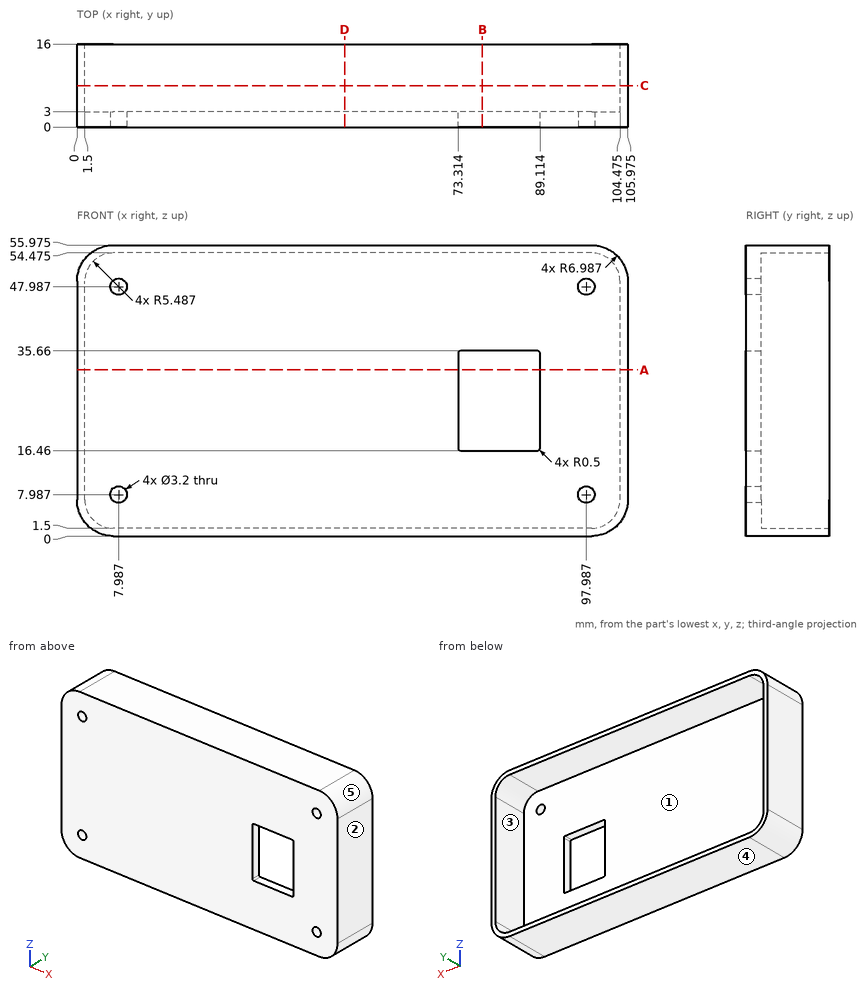
Design review of the part shown in the three views and the two pictorial views. Dimensions are in mm from the part's minimum x, y and z. A direction names the side the tool comes from. Coordinates: 2 decimals unless noted, no trailing zeros. Order: outer loops, then holes, each group sorted by start corner. A loop starts at its lowest first (then second) coordinate and runs counter-clockwise, first axis right, second up. Notation, with made-up numbers: (55.25, 55.25) - (98.25, 55.25) arc R25 cw to (98.25, 83.25) - close; hole circle Ø8 at (13.25, 28.5). An arc over 180 degrees is marked (long way). One line per question, with ' | ' between items.
Q1. For the marked faces 1 and 2, list the 3-axis set-ups (+Z, -Z, +X, -X, +Y, -Y) from which the entire face can be reached by the end or side of a thin tool; tool diameter is ignored.
Answer key:
face 1: +Y | face 2: +Z, -Z, +X, +Y, -Y
Q2. The part is to be moulded in two halves that separate along X. For the marked faces 3, 4 and 5, say which applies: +X half, -X half, draft (parallel to the pull), parting line (faces both ways), or undercut.
Answer key:
face 3: undercut | face 4: draft | face 5: +X half
Q3. Consider section B-B, the plane x = 78. Give the boundary of the cut face in (y, z) (1 decimal), then the cut area to 3 significant figures.
Answer key:
outline: (0, 0) - (16, 0) - (16, 1.5) - (3, 1.5) - (3, 16.5) - (0, 16.5) - close; (0, 35.7) - (3, 35.7) - (3, 54.5) - (16, 54.5) - (16, 56) - (0, 56) - close | area: 149 mm2
Q4. Clearance check with flat-ended pins moving along their axes: pin 1 Ø1.9 at (x, z) = (97.99, 7.99) entering from -Y; pin 2 Ø2 at (x, z) = (92, 9) entering from +Y. State where each tip first meets the part, or that it passes through.
Answer key:
pin 1: passes through | pin 2: stops at y = 3
Q5. Consider section D-D, the plane x = 51.5. Give the boundary of the cut face in (y, z) (1 decimal), then the cut area to 3 significant figures.
Answer key:
outline: (0, 0) - (16, 0) - (16, 1.5) - (3, 1.5) - (3, 54.5) - (16, 54.5) - (16, 56) - (0, 56) - close | area: 207 mm2
Q6. To check wall thickness, follow line 1 along X through (y, z) = (0.5, 28) (1 decimal); line 2 along X through (y, z) = (14.25, 36.5) (1 decimal); line 3 along Z through (x, y) = (66, 9) (1 decimal). State the ranges of each line that lie inside material, in increasing order.
Answer key:
line 1: x = 0 to 73.3, 89.1 to 106 | line 2: x = 0 to 1.5, 104.5 to 106 | line 3: z = 0 to 1.5, 54.5 to 56
Q7. Consider section C-C, the plane y = 8. Give the boundary of the cut face in (x, z) (1 decimal).
Answer key:
outline: (0, 7) arc R7 ccw to (7, 0) - (99, 0) arc R7 ccw to (106, 7) - (106, 49) arc R7 ccw to (99, 56) - (7, 56) arc R7 ccw to (0, 49) - close; hole (1.5, 7) arc R5.5 ccw to (7, 1.5) - (99, 1.5) arc R5.5 ccw to (104.5, 7) - (104.5, 49) arc R5.5 ccw to (99, 54.5) - (7, 54.5) arc R5.5 ccw to (1.5, 49) - close
Q8. Consider section A-A, the plane z = 32. Give the boundary of the cut face in (x, y) (1 decimal).
Answer key:
outline: (0, 0) - (73.3, 0) - (73.3, 3) - (1.5, 3) - (1.5, 16) - (0, 16) - close; (89.1, 0) - (106, 0) - (106, 16) - (104.5, 16) - (104.5, 3) - (89.1, 3) - close
